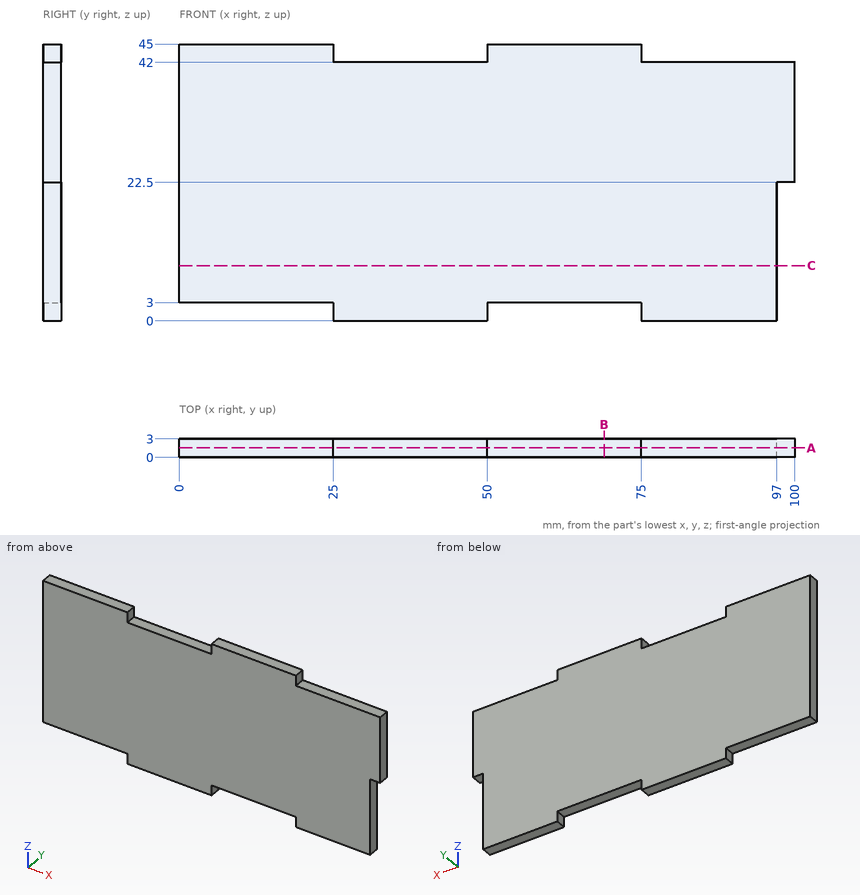
For this review, use the dimensioned drawing (mm, ordinates from the lowest corner) and the shaded views. Give positions to 0.01 mm unless a question says otherwise; leave off trailing zeros. Loops run counter-clockwise (first coordinate to the right, second up) from the corner with the lowest first, then second, coordinate; pieces in that order, holes last.
Item 1: Insertion check: pin 1 (1.5 mm diameter, centred on x = 60.5, y = 2, fed in from -Z); pin 2 (0.9 mm diameter, centred on y = 1, z = 1.5, fed in from -X); pin 3 (0.9 mm diameter, centred on x = 90.5, y = 2, fed in from +Z). Each pin has a flat end and moves straight along its axis. Give the tip position at first contact, or say it passes through.
Item 2: Take a section at C-C, the plane z = 9. State the section outline as (x, y) points, and give its area (3 significant figures).
Item 3: Take a section at B-B, the plane x = 69. State the section outline as (y, z) points.
Item 4: For line 1 along Z through (x, y) = (80, 2.6); line 2 along Z through (x, y) = (13, 2.15); line 3 along X through (y, z) = (1.9, 16), list the stretches that pass through material, from the lowest coordinate up.
Item 5: Take a section at A-A, the plane y = 1.55. State the section outline as (x, z) points, and give its area (3 significant figures).
Calculated:
1. pin 1: stops at z = 3
1. pin 2: stops at x = 25
1. pin 3: stops at z = 42
2. outline: (0, 0) - (97, 0) - (97, 3) - (0, 3) - close
2. area: 291 mm2
3. outline: (0, 3) - (3, 3) - (3, 45) - (0, 45) - close
4. line 1: z = 0 to 42
4. line 2: z = 3 to 45
4. line 3: x = 0 to 97
5. outline: (0, 3) - (25, 3) - (25, 0) - (50, 0) - (50, 3) - (75, 3) - (75, 0) - (97, 0) - (97, 22.5) - (100, 22.5) - (100, 42) - (75, 42) - (75, 45) - (50, 45) - (50, 42) - (25, 42) - (25, 45) - (0, 45) - close
5. area: 4,130 mm2
